The listing builds one solid part. Answer for the finished solid, in the listing's coordinates (mm). Round coordinates to 2 decimals unless told otherwise and drop trailing zeros. Write each loop counter-clockwise with the first axis right and the second up, starting at its lowest first coordinate (ties: lowest second). Pieces come first, ordered by that corner, then holes.
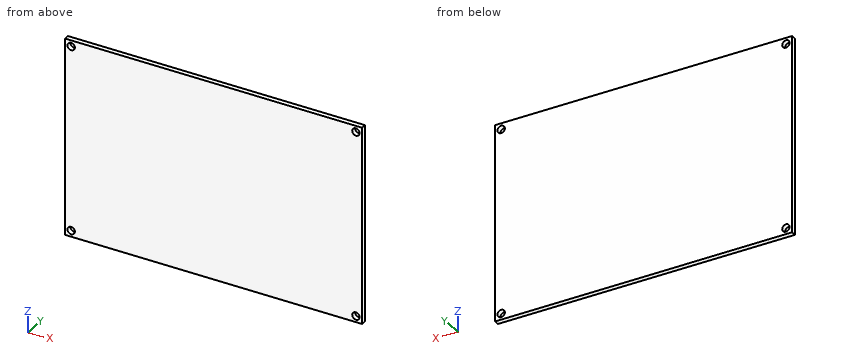
Autodesk Inventor part; units mm, degrees
sketch "Эскиз1" plane through (0, 0, 0) normal (0, 1, 0) x (-1, 0, 0)
  line L0 (60, 40) -> (-60, 40)
  line L1 (-60, 40) -> (-60, -40)
  line L2 (-60, -40) -> (60, -40)
  line L3 (60, -40) -> (60, 40)
  line L4 (60, 40) -> (-60, -40) construction
  line L5 (-60, 40) -> (60, -40) construction
  point P0 (0, 0)
  dimension "d0" = 120
  dimension "d1" = 80
extrude "Выдавливание1" add sketch "Эскиз1" along normal blind 2
sketch "Эскиз2" plane through (0, 2, 0) normal (0, 1, 0) x (1, 0, 0)
  circle A0 centre (-57.5, 37.5) radius 1.5
  line L0 (-60, 40) -> (-60, -40)
  line L1 (60, 40) -> (-60, 40)
  line L2 (0, 56) -> (0, -56) construction
  line L3 (84, 0) -> (-84, 0) construction
  circle A1 centre (57.5, 37.5) radius 1.5
  circle A2 centre (-57.5, -37.5) radius 1.5
  circle A3 centre (57.5, -37.5) radius 1.5
  dimension "d4" = 3
  dimension "d5" = 2.5
  dimension "d6" = 2.5
extrude "Выдавливание2" cut sketch "Эскиз2" against normal up to next
properties part number "Плата"
1. Section A-A on z = 37.5 is taken. Determine the outline of the cut face in (x, y), plus the area to 3 significant figures.
Geometry says:
outline: (-60, 0) - (-59, 0) - (-59, 2) - (-60, 2) - close; (-56, 0) - (56, 0) - (56, 2) - (-56, 2) - close; (59, 0) - (60, 0) - (60, 2) - (59, 2) - close
area: 228 mm2
2. Straight lines are drawn through the part: line 1 along X through (y, z) = (1.1, 37.5); line 2 along Z through (x, y) = (-57.5, 0.7). For each, find the intervals that lie inside material, in ascending order.
Geometry says:
line 1: x = -60 to -59, -56 to 56, 59 to 60
line 2: z = -40 to -39, -36 to 36, 39 to 40
3. Section B-B on x = -57.5 is taken. Determine the outline of the cut face in (y, z), plus the area to 3 significant figures.
Geometry says:
outline: (0, -40) - (2, -40) - (2, -39) - (0, -39) - close; (0, -36) - (2, -36) - (2, 36) - (0, 36) - close; (0, 39) - (2, 39) - (2, 40) - (0, 40) - close
area: 148 mm2
4. Given pin 1 (2.5 mm diameter, centred on x = -57.5, z = -37.5, fed in from +Y), flat-ended and moving along its own axis, determine where the tip first touches the part or whether it passes through.
Geometry says:
pin 1: passes through
